Can you work these out from the model? Positions are in its coordinate system, mm. A direction names the side the tool comes from. Give positions to 0.01 mm unless a question says otherwise; leave off trailing zeros. Write each loop counter-clockwise with the first axis right and the second up, starting at its lowest first coordinate (ties: lowest second). Pieces come first, ordered by that corner, then holes.
1. Suppose I cut it at A-A (y = 36). Please give me the cut outline in (x, z).
2. Suppose I cut it at B-B (y = 5.5). Please give me the cut outline in (x, z).
3. On a 3-axis mill with a long thin cutter (end or side, diameter ignored), from which of +Z, -Z, +X, -X, +Y, -Y can I reach the whole of each face in a straight line? I mean faces 1 (the cylindrical face through (-18.207, -35.616, 7.395)), 2 (the flat face through (-40.65, 10.58, 7.4)), 3 (the flat face through (26.67, -32.455, 7.395)). Say none if no direction works.
4. Thinking about a two-plate mould opening in X: for faces 4 (the flat face through (-40.7, -10.6, 7.4)), 5 (the flat face through (0, -44, 7)), 6 (the cylindrical face through (-28.25, 28.32, 7.4)), which applies, pulls with the +X half, pulls with the -X half, needs draft (parallel to the pull), parting line crosses it, or undercut?
5. I'm going to push flat-ended pins straight in: pin 1 (2 mm diameter, centred on y = 22, z = 13.5, fed in from +X); pin 2 (2 mm diameter, centred on x = -41.5, z = 8.5, fed in from +Y); pin 3 (4.5 mm diameter, centred on y = 41.5, z = 8, fed in from -X). Where does each tip first touch, or does it pass through?
6. If I drill on probe 1 along X at (y, z) = (-27.5, 1); probe 2 along X at (y, z) = (-27, 10.5); probe 3 along Y at (x, z) = (36.5, 10.25), over which ranges is the centre line in solid material (lowest first)?
```python
from build123d import *

# Parameters (mm, degrees)
SKETCH_1_R               = 40
EXTRUDE_1_DEPTH          = 15
SKETCH_2_W               = 4.077896861
SKETCH_2_H               = 4.995131446
EXTRUDE_2_DEPTH          = 15
PATTERN_CIRCULAR_1_COUNT = 20


with BuildPart() as part:
    # Sketch 1 → Extrude 1 (new body)
    with BuildSketch(Plane.XY):
        Circle(SKETCH_1_R)
    extrude(amount=EXTRUDE_1_DEPTH)

    # Sketch 2 → Extrude 2 (add)
    with BuildSketch(Plane.XY):
        with Locations((41.96105157, 0.002434277)):
            Rectangle(SKETCH_2_W, SKETCH_2_H)
    extrude_2 = extrude(amount=EXTRUDE_2_DEPTH)

    # Pattern Circular 1: Extrude 2 ×20 about axis
    pattern_circular_1_axis = Axis((0, 0, 0), (0, 0, 1))
    for i in range(1, PATTERN_CIRCULAR_1_COUNT):
        add(extrude_2.rotate(pattern_circular_1_axis, i * 360 / PATTERN_CIRCULAR_1_COUNT))


solid = part.part
```
Checks:
1. outline: (-25.31, 0) - (-23.07, 0) - (-23.07, 15) - (-25.31, 15) - close; (-17.44, 0) - (17.44, 0) - (17.44, 15) - (-17.44, 15) - close; (23.07, 0) - (25.31, 0) - (25.31, 15) - (23.07, 15) - close
2. outline: (-39.62, 0) - (39.62, 0) - (39.62, 15) - (-39.62, 15) - close
3. face 1: +Z, -Z
3. face 2: +Z, -Z, -X
3. face 3: +Z, -Z, +X
4. face 4: pulls with the -X half
4. face 5: needs draft
4. face 6: undercut
5. pin 1: stops at x = 35.9
5. pin 2: stops at y = 15.97
5. pin 3: stops at x = -15.97
6. probe 1: x = -34.41 to -33.6, -29.05 to 29.05, 33.61 to 34.41
6. probe 2: x = -34.77 to -32.91, -29.51 to 29.51, 32.92 to 34.77
6. probe 3: y = -24.62 to -23.43, -16.36 to 16.36, 23.43 to 24.62
